```python
from build123d import *

# Parameters (mm, degrees)
F0_R     = 2.25
F1_DEPTH = 55
F2_DEPTH = 5
F3_R     = 1.65
F4_DEPTH = 10


with BuildPart() as f1:
    # F0 (on Top) → F1 (new body)
    with BuildSketch(Plane.XY):
        Polygon((4, -2.309401), (4, 2.309401), (0, 4.618802), (-4, 2.309401), (-4, -2.309401), (0, -4.618802), align=None)
        Circle(F0_R, mode=Mode.SUBTRACT)
        Circle(F0_R)
    extrude(amount=F1_DEPTH)

    # F0 (on Top) → F2 (join)
    with BuildSketch(Plane.XY):
        Circle(F0_R)
    extrude(amount=-F2_DEPTH)

    # F3 (on face) → F4 (cut)
    with BuildSketch(Plane.XY.offset(55)):
        Circle(F3_R)
    extrude(amount=-F4_DEPTH, mode=Mode.SUBTRACT)


solid = f1.part
```
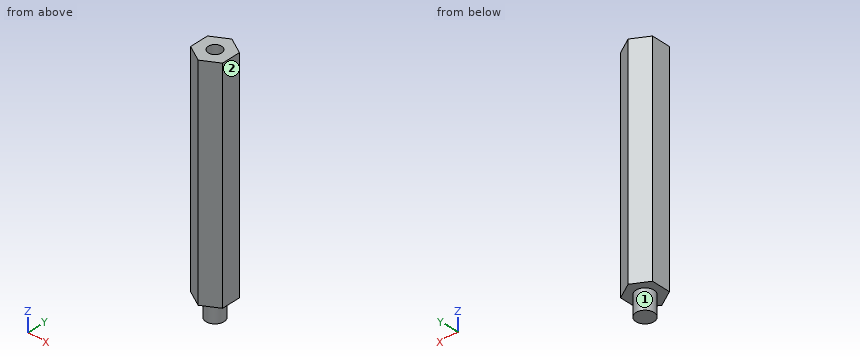
Geometry: final body of the model. Coordinates: model frame, mm. Face numbers are marked on the shaded views. A direction names the side the tool comes from. Coordinates: 2 decimals unless noted, no trailing zeros. Order: outer loops, then holes, each group sorted by start corner. A loop starts at its lowest first (then second) coordinate and runs counter-clockwise, first axis right, second up. Notation, with made-up numbers: (-9.75, -39.5) -> (25.25, -39.5) arc R19 ccw to (25.25, -19.5) -> close; hole circle Ø9 at (69.25, -20). An arc over 180 degrees is marked (long way). Answer in a Markdown table with one row per item.
Item 1: Access query for the marked faces 1 and 2. Directions: +Z, -Z, +X, -X, +Y, -Y. A direction counts if a zero-diameter tool reaches every point of the face in a straight line with its end or side. Return the directions, or none.
Return value:
| item | result |
|---|---|
| face 1 | -Z |
| face 2 | +Z, -Z, +X, +Y, -Y |
Item 2: Contact query for flat-ended pins moving along their axis: P1, Ø1.5, axis at x = 2, y = -3.5, coming from the +Z side; P2, Ø3, axis at x = 0, y = 0, coming from the +Z side; P3, Ø2, axis at x = -3, z = 40, coming from the +Y side; P4, Ø2, axis at x = 2.5, y = -2.5, coming from the -Z side. Output: stop coordinate, or through.
Return value:
| item | result |
|---|---|
| P1 | stops at z = 55 |
| P2 | stops at z = 45 |
| P3 | stops at y = 3.46 |
| P4 | stops at z = 0 |
Item 3: Ray query, L1, parallel to Y at x = 0, z = 52; L2, parallel to Z at x = -0.5, y = -4; L3, parallel to X at y = 1.25, z = 48. Return the intervals inside material, ascending.
Return value:
| item | result |
|---|---|
| L1 | y = -4.62 to -1.65, 1.65 to 4.62 |
| L2 | z = 0 to 55 |
| L3 | x = -4 to -1.08, 1.08 to 4 |
Item 4: Section C-C on z = 21.5. Output: boundary loops of the cut face in (x, y).
Return value:
| item | result |
|---|---|
| outline | (-4, -2.31) -> (0, -4.62) -> (4, -2.31) -> (4, 2.31) -> (0, 4.62) -> (-4, 2.31) -> close |
Item 5: Section B-B on y = 0. Output: boundary loops of the cut face in (x, z), plus the area to 4 significant figures.
Return value:
| item | result |
|---|---|
| outline | (-4, 0) -> (-2.25, 0) -> (-2.25, -5) -> (2.25, -5) -> (2.25, 0) -> (4, 0) -> (4, 55) -> (1.65, 55) -> (1.65, 45) -> (-1.65, 45) -> (-1.65, 55) -> (-4, 55) -> close |
| area | 429.5 mm² |
Item 6: Section A-A on z = 51.5. Output: boundary loops of the cut face in (x, y).
Return value:
| item | result |
|---|---|
| outline | (-4, -2.31) -> (0, -4.62) -> (4, -2.31) -> (4, 2.31) -> (0, 4.62) -> (-4, 2.31) -> close; hole circle Ø3.3 at (0, 0) |
Item 7: Section D-D on x = -1. Output: boundary loops of the cut face in (y, z).
Return value:
| item | result |
|---|---|
| outline | (-4.04, 0) -> (-2.02, 0) -> (-2.02, -5) -> (2.02, -5) -> (2.02, 0) -> (4.04, 0) -> (4.04, 55) -> (1.31, 55) -> (1.31, 45) -> (-1.31, 45) -> (-1.31, 55) -> (-4.04, 55) -> close |
